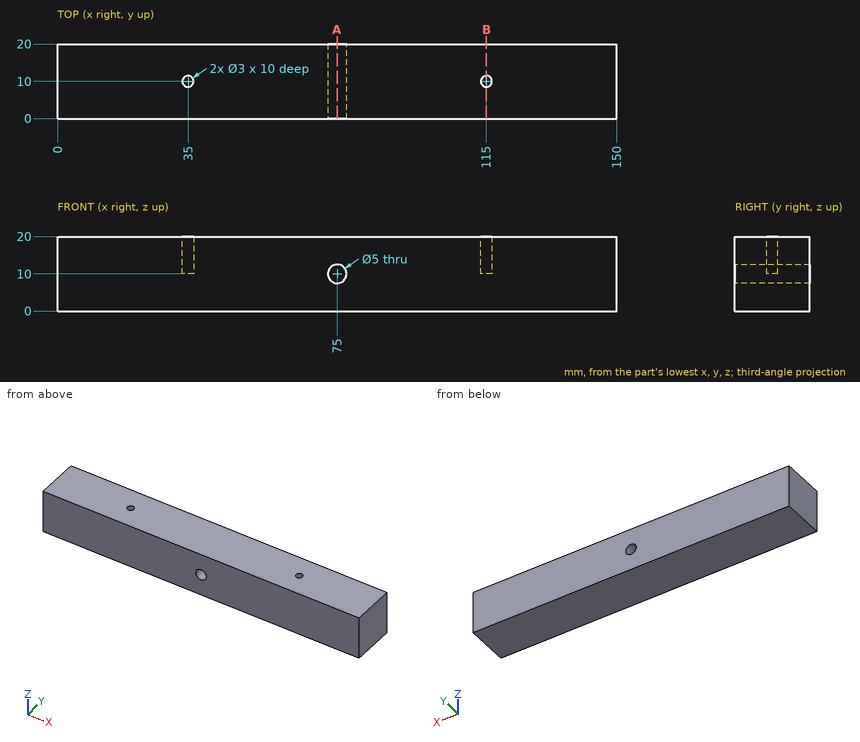
For this review, use the dimensioned drawing (mm, ordinates from the lowest corner) and the shaded views. Coordinates: 2 decimals unless noted, no trailing zeros. Loops run counter-clockwise (first coordinate to the right, second up) from the corner with the lowest first, then second, coordinate; pieces in that order, holes last.
1. For line 1 (Z direction, x = 75, y = 8.5); line 2 (Y direction, x = 35, z = 16); line 3 (X direction, y = 15, z = 11.5), list the stretches that pass through material, from the lowest coordinate up.
2. Add section A-A, the plane x = 75. Give the boundary of the cut face in (y, z).
3. Insertion check: P1, Ø8, axis at y = 17, z = 8.5, coming from the -X side; P2, Ø2.5, axis at x = 35, y = 10, coming from the +Z side; P3, Ø3, axis at x = 75, z = 10, coming from the +Y side. Each pin has a flat end and moves straight along its axis. Give the tip position at first contact, or say it passes through.
4. Add section B-B, the plane x = 115. Give the boundary of the cut face in (y, z), then the cut area to 3 significant figures.
Result:
1. line 1: z = 0 to 7.5, 12.5 to 20
1. line 2: y = 0 to 8.5, 11.5 to 20
1. line 3: x = 0 to 73, 77 to 150
2. outline: (0, 0) - (20, 0) - (20, 7.5) - (0, 7.5) - close; (0, 12.5) - (20, 12.5) - (20, 20) - (0, 20) - close
3. P1: stops at x = 0
3. P2: stops at z = 10
3. P3: passes through
4. outline: (0, 0) - (20, 0) - (20, 20) - (11.5, 20) - (11.5, 10) - (8.5, 10) - (8.5, 20) - (0, 20) - close
4. area: 370 mm2
